Answer from the drawing. Dimensions are ordinates in mm from the lowest x, y and z of the part. A direction names the side the tool comes from. Coordinates: 2 decimals unless noted, no trailing zeros. Order: outer loops, then holes, each group sorted by start corner. A loop starts at its lowest first (then second) coordinate and runs counter-clockwise, first axis right, second up. Notation, with made-up numbers: (68.25, 70.5) -> (105.25, 70.5) arc R30 ccw to (105.25, 102.5) -> close; hole circle Ø4 at (-1, 1). An arc over 180 degrees is marked (long way). Answer in a Markdown table with one row per item.
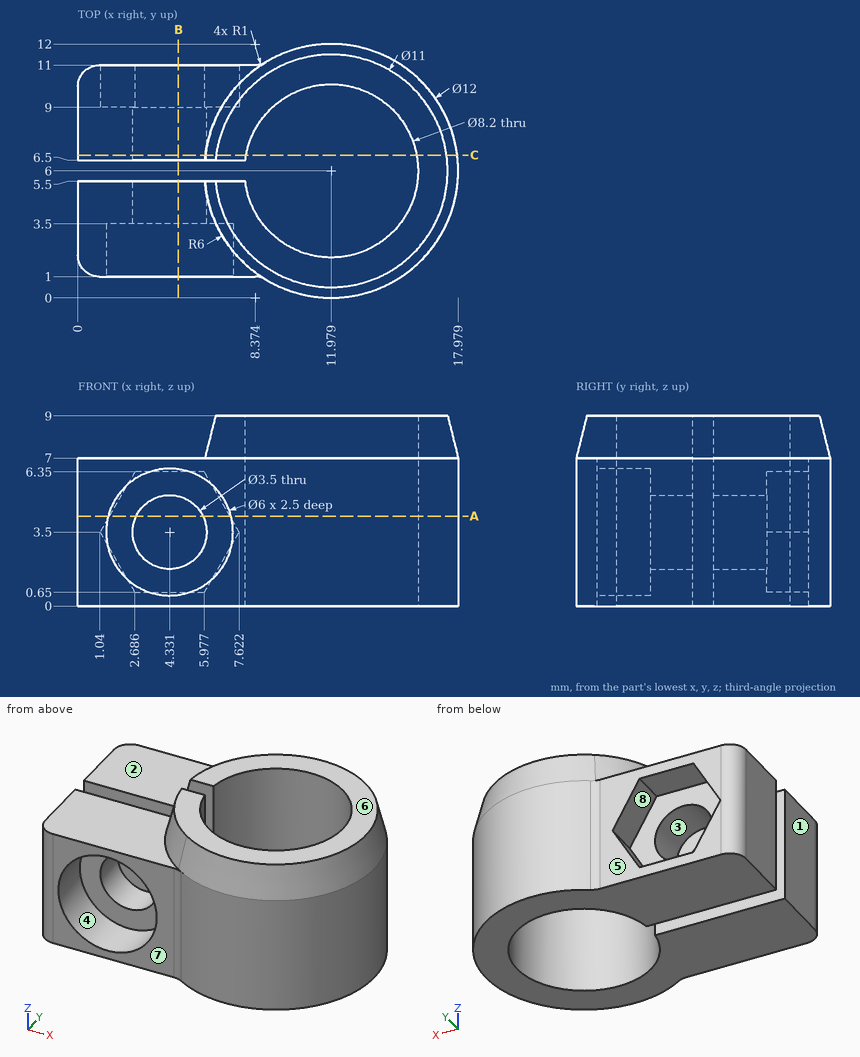
(1) Find the intervals of material crossed by line 1 along Y through (x, z) = (5, 1.5); line 2 along X through (y, z) = (2.75, 5.25) (1 decimal); line 3 along X through (y, z) = (3, 5.5) (1 decimal), in increasing order. Write a range as from..to.
Check values:
| item | result |
|---|---|
| line 1 | 3.5..5.5, 6.5..9 |
| line 2 | 0..1.9, 6.8..9.5, 14.5..17 |
| line 3 | 0..2.1, 6.6..9.2, 14.8..17.2 |
(2) A cutting plane is placed at C-C, the plane y = 6.75. Count the separate pieces of the cut face and the enclosed holes in it.
Check values:
| item | result |
|---|---|
| separate pieces | 2 |
| enclosed holes | 1 |
(3) A cutting plane is placed at B-B, the plane x = 4.75. Determine the outline of the cut face in (y, z).
Check values:
| item | result |
|---|---|
| outline | (1, 0) -> (5.5, 0) -> (5.5, 1.8) -> (3.5, 1.8) -> (3.5, 0.53) -> (1, 0.53) -> close; (1, 6.47) -> (3.5, 6.47) -> (3.5, 5.2) -> (5.5, 5.2) -> (5.5, 7) -> (1, 7) -> close; (6.5, 0) -> (11, 0) -> (11, 0.65) -> (9, 0.65) -> (9, 1.8) -> (6.5, 1.8) -> close; (6.5, 5.2) -> (9, 5.2) -> (9, 6.35) -> (11, 6.35) -> (11, 7) -> (6.5, 7) -> close |
(4) Flat-ended cylindrical pins translate along their axes: pin 1 (1.4 mm diameter, centred on x = 5, y = 8.5, fed in from +Z); pin 2 (4 mm diameter, centred on x = 4.33, z = 3.5, fed in from +Y); pin 3 (4.5 mm diameter, centred on x = 4.33, z = 3.5, fed in from -Y). Find the tip coordinate at first contact, or state that the pin passes through.
Check values:
| item | result |
|---|---|
| pin 1 | z = 7 |
| pin 2 | y = 9 |
| pin 3 | y = 3.5 |
(5) Which of the six approach directions +Z, -Z, +X, -X, +Y, -Y give full straight-line access (tool end or side, diameter ignored) to the marked faces 4, 5, 6, 7 and 8?
Check values:
| item | result |
|---|---|
| face 4 | -Y |
| face 5 | +Z, -Z, -X, +Y |
| face 6 | +Z, +X, -X, +Y, -Y |
| face 7 | +Z, -Z, -X, -Y |
| face 8 | +Y |
(6) For a pull along X with two mould halves and no side action, classify the marked faces 1, 2 and 3 as released by +X, released by -X, zero draft, split by the parting line, or undercut.
Check values:
| item | result |
|---|---|
| face 1 | released by -X |
| face 2 | zero draft |
| face 3 | undercut |
(7) A cutting plane is placed at A-A, the plane z = 4.25. Determine the outline of the cut face in (x, y).
Check values:
| item | result |
|---|---|
| outline | (0, 2) arc R1 ccw to (1, 1) -> (1.43, 1) -> (1.43, 3.5) -> (2.75, 3.5) -> (2.75, 5.5) -> (0, 5.5) -> close; (0, 6.5) -> (2.75, 6.5) -> (2.75, 9) -> (1.47, 9) -> (1.47, 11) -> (1, 11) arc R1 ccw to (0, 10) -> close; (5.91, 3.5) -> (7.24, 3.5) -> (7.24, 1) -> (8.37, 1) arc R1 cw to (8.89, 0.86) arc R6 ccw (long way) to (8.89, 11.14) arc R1 cw to (8.37, 11) -> (7.19, 11) -> (7.19, 9) -> (5.91, 9) -> (5.91, 6.5) -> (7.91, 6.5) arc R4.1 cw (long way) to (7.91, 5.5) -> (5.91, 5.5) -> close |
